Design review of the part built by this model. Coordinates are the model's own, in mm. A direction names the side the tool comes from. Give positions to 0.01 mm unless a question says otherwise; leave off trailing zeros. Write each loop counter-clockwise with the first axis right and the second up, starting at its lowest first coordinate (ties: lowest second). Pieces come first, ordered by that corner, then holes.
```python
from build123d import *

# Parameters (mm, degrees)
F0_W     = 482.6
F0_H     = 50.8
F0_W_2   = 50.8
F0_W_3   = 152.4
F0_H_2   = 101.6
F0_W_4   = 482.6000000003
F0_H_3   = 152.4
F0_W_5   = 381.0000000003
F0_W_6   = 151.9448201656
F0_H_4   = 76.2
F0_W_7   = 51.7103596687
F0_H_5   = 177.8
F0_H_6   = 279.4
F0_W_8   = 380.9999999997
F1_DEPTH = 50.8


with BuildPart() as f1:
    # F0 (on Front) → F1 (new body)
    with BuildSketch(Plane.XZ):
        with Locations((-977.9, 101.6)):
            Rectangle(F0_W, F0_H)
        with Locations((-711.2, 101.6)):
            Rectangle(F0_W_2, F0_H)
        Polygon((-685.8, 76.2), (-736.6, 76.2), (-736.6, -76.2), (-685.8, -76.2), (-685.8, 0), align=None)
        with Locations((-609.6, 101.6)):
            Rectangle(F0_W_3, F0_H)
        with Locations((-711.2, 177.8)):
            Rectangle(F0_W_2, F0_H_2)
        with Locations((-977.9000000001, -101.6)):
            Rectangle(F0_W_4, F0_H)
        with Locations((-711.2, -101.6)):
            Rectangle(F0_W_2, F0_H)
        with Locations((-508, 101.6)):
            Rectangle(F0_W_2, F0_H)
        with Locations((-609.6, -101.6)):
            Rectangle(F0_W_3, F0_H)
        with Locations((-711.2, -177.8)):
            Rectangle(F0_W_2, F0_H_2)
        with Locations((-508, 203.2)):
            Rectangle(F0_W_2, F0_H_3)
        with Locations((-508, -101.6)):
            Rectangle(F0_W_2, F0_H)
        with Locations((-508, 304.8)):
            Rectangle(F0_W_2, F0_H)
        with Locations((-723.9000000001, 304.8)):
            Rectangle(F0_W_5, F0_H)
        with Locations((-508, -203.2)):
            Rectangle(F0_W_2, F0_H_3)
        with Locations((-406.6275899172, 304.8)):
            Rectangle(F0_W_6, F0_H)
        with Locations((-508, 368.3)):
            Rectangle(F0_W_2, F0_H_4)
        with Locations((-723.9000000001, -304.8)):
            Rectangle(F0_W_5, F0_H)
        with Locations((-508, -304.8)):
            Rectangle(F0_W_2, F0_H)
        with Locations((-304.8, 304.8)):
            Rectangle(F0_W_7, F0_H)
        with Locations((-406.6275899172, -304.8)):
            Rectangle(F0_W_6, F0_H)
        with Locations((-508, -368.3)):
            Rectangle(F0_W_2, F0_H_4)
        with Locations((-202.9724100828, 304.8)):
            Rectangle(F0_W_6, F0_H)
        with Locations((-304.8, 419.1)):
            Rectangle(F0_W_7, F0_H_5)
        with Locations((-304.8, -304.8)):
            Rectangle(F0_W_7, F0_H)
        with Locations((-101.6, 304.8)):
            Rectangle(F0_W_2, F0_H)
        with Locations((-202.9724100828, -304.8)):
            Rectangle(F0_W_6, F0_H)
        with Locations((-304.8, -419.1)):
            Rectangle(F0_W_7, F0_H_5)
        Polygon((-76.2, 330.2), (-76.2, 279.4), (-2e-10, 279.4), (76.2, 279.4), (76.2, 330.2), align=None)
        with Locations((-101.6, 469.9)):
            Rectangle(F0_W_2, F0_H_6)
        with Locations((-101.6, -304.8)):
            Rectangle(F0_W_2, F0_H)
        with Locations((101.6, 304.8)):
            Rectangle(F0_W_2, F0_H)
        Polygon((-3e-10, -279.4), (-76.2, -279.4), (-76.2, -330.2), (76.2, -330.2), (76.2, -279.4), align=None)
        with Locations((-101.6, -469.9)):
            Rectangle(F0_W_2, F0_H_6)
        with Locations((203.2, 304.8)):
            Rectangle(F0_W_3, F0_H)
        with Locations((101.6, 469.9)):
            Rectangle(F0_W_2, F0_H_6)
        with Locations((101.6, -304.8)):
            Rectangle(F0_W_2, F0_H)
        with Locations((508, 101.6)):
            Rectangle(F0_W_2, F0_H)
        with Locations((304.8, 304.8)):
            Rectangle(F0_W_2, F0_H)
        with Locations((203.2, -304.8)):
            Rectangle(F0_W_3, F0_H)
        with Locations((101.6, -469.9)):
            Rectangle(F0_W_2, F0_H_6)
        with Locations((609.6, 101.6)):
            Rectangle(F0_W_3, F0_H)
        with Locations((508, 203.2)):
            Rectangle(F0_W_2, F0_H_3)
        with Locations((406.4, 304.8)):
            Rectangle(F0_W_3, F0_H)
        with Locations((304.8, 419.1)):
            Rectangle(F0_W_2, F0_H_5)
        with Locations((508, -101.6)):
            Rectangle(F0_W_2, F0_H)
        with Locations((304.8, -304.8)):
            Rectangle(F0_W_2, F0_H)
        with Locations((711.2, 101.6)):
            Rectangle(F0_W_2, F0_H)
        Polygon((736.6, 76.2), (685.8, 76.2), (685.8, 0), (685.8, -76.2), (736.6, -76.2), align=None)
        with Locations((508, 304.8)):
            Rectangle(F0_W_2, F0_H)
        with Locations((609.6, -101.6)):
            Rectangle(F0_W_3, F0_H)
        with Locations((508, -203.2)):
            Rectangle(F0_W_2, F0_H_3)
        with Locations((406.4, -304.8)):
            Rectangle(F0_W_3, F0_H)
        with Locations((304.8, -419.1)):
            Rectangle(F0_W_2, F0_H_5)
        with Locations((977.9000000001, 101.6)):
            Rectangle(F0_W_4, F0_H)
        with Locations((711.2, 177.8)):
            Rectangle(F0_W_2, F0_H_2)
        with Locations((723.8999999999, 304.8)):
            Rectangle(F0_W_8, F0_H)
        with Locations((508, 368.3)):
            Rectangle(F0_W_2, F0_H_4)
        with Locations((711.2, -101.6)):
            Rectangle(F0_W_2, F0_H)
        with Locations((508, -304.8)):
            Rectangle(F0_W_2, F0_H)
        with Locations((977.9, -101.6)):
            Rectangle(F0_W, F0_H)
        with Locations((711.2, -177.8)):
            Rectangle(F0_W_2, F0_H_2)
        with Locations((723.8999999999, -304.8)):
            Rectangle(F0_W_8, F0_H)
        with Locations((508, -368.3)):
            Rectangle(F0_W_2, F0_H_4)
        with Locations((-304.8, 203.2)):
            Rectangle(F0_W_7, F0_H_3)
        with Locations((-101.6, 203.2)):
            Rectangle(F0_W_2, F0_H_3)
        with Locations((101.6, 203.2)):
            Rectangle(F0_W_2, F0_H_3)
        with Locations((304.8, 203.2)):
            Rectangle(F0_W_2, F0_H_3)
        Polygon((330.2, 76.2), (279.4, 76.2), (279.4, 0), (304.8, 0), (330.2, 0), align=None)
        Polygon((304.8, 0), (279.4, 0), (279.4, -76.2), (330.2, -76.2), (330.2, 0), align=None)
        with Locations((304.8, -101.6)):
            Rectangle(F0_W_2, F0_H)
        with Locations((304.8, -203.2)):
            Rectangle(F0_W_2, F0_H_3)
        with Locations((304.8, 101.6)):
            Rectangle(F0_W_2, F0_H)
        Polygon((533.4, 76.2), (482.6, 76.2), (482.6, 0), (508, 0), (533.4, 0), align=None)
        Polygon((508, 0), (482.6, 0), (482.6, -76.2), (533.4, -76.2), (533.4, 0), align=None)
        with Locations((101.6, -203.2)):
            Rectangle(F0_W_2, F0_H_3)
        with Locations((101.6, -101.6)):
            Rectangle(F0_W_2, F0_H)
        Polygon((101.6, 0), (76.2, 0), (76.2, -76.2), (127, -76.2), (127, 0), align=None)
        Polygon((127, 76.2), (76.2, 76.2), (76.2, 0), (101.6, 0), (127, 0), align=None)
        with Locations((101.6, 101.6)):
            Rectangle(F0_W_2, F0_H)
        with Locations((-101.6, 101.6)):
            Rectangle(F0_W_2, F0_H)
        Polygon((-76.2, 76.2), (-127, 76.2), (-127, 0), (-101.6, 0), (-76.2, 0), align=None)
        Polygon((-101.6, 0), (-127, 0), (-127, -76.2), (-76.2, -76.2), (-76.2, 0), align=None)
        with Locations((-101.6, -101.6)):
            Rectangle(F0_W_2, F0_H)
        with Locations((-101.6, -203.2)):
            Rectangle(F0_W_2, F0_H_3)
        with Locations((-304.8, -203.2)):
            Rectangle(F0_W_7, F0_H_3)
        with Locations((-304.8, -101.6)):
            Rectangle(F0_W_7, F0_H)
        Polygon((-304.8, 0), (-330.6551798344, 0), (-330.6551798344, -76.2), (-278.9448201656, -76.2), (-278.9448201656, 0), align=None)
        Polygon((-278.9448201656, 76.2), (-330.6551798344, 76.2), (-330.6551798344, 0), (-304.8, 0), (-278.9448201656, 0), align=None)
        with Locations((-304.8, 101.6)):
            Rectangle(F0_W_7, F0_H)
        Polygon((-482.6, 76.2), (-533.4, 76.2), (-533.4, 0), (-508, 0), (-482.6, 0), align=None)
        Polygon((-508, 0), (-533.4, 0), (-533.4, -76.2), (-482.6, -76.2), (-482.6, 0), align=None)
        with Locations((-406.6275899172, 101.6)):
            Rectangle(F0_W_6, F0_H)
        with Locations((-202.9724100828, 101.6)):
            Rectangle(F0_W_6, F0_H)
        Polygon((-76.2, 127), (-76.2, 76.2), (76.2, 76.2), (76.2, 127), (0, 127), align=None)
        with Locations((203.2, 101.6)):
            Rectangle(F0_W_3, F0_H)
        with Locations((406.4, 101.6)):
            Rectangle(F0_W_3, F0_H)
        with Locations((406.4, -101.6)):
            Rectangle(F0_W_3, F0_H)
        with Locations((203.2, -101.6)):
            Rectangle(F0_W_3, F0_H)
        Polygon((76.2, -76.2), (-76.2, -76.2), (-76.2, -127), (-3e-10, -127), (76.2, -127), align=None)
        with Locations((-202.9724100828, -101.6)):
            Rectangle(F0_W_6, F0_H)
        with Locations((-406.6275899172, -101.6)):
            Rectangle(F0_W_6, F0_H)
    extrude(amount=F1_DEPTH)


solid = f1.part
```
(1) Consider section C-C, the plane x = -609. Give the boundary of the cut face in (y, z).
Resolved:
outline: (-50.8, -330.2) - (0, -330.2) - (0, -279.4) - (-50.8, -279.4) - close; (-50.8, -127) - (0, -127) - (0, -76.2) - (-50.8, -76.2) - close; (-50.8, 76.2) - (0, 76.2) - (0, 127) - (-50.8, 127) - close; (-50.8, 279.4) - (0, 279.4) - (0, 330.2) - (-50.8, 330.2) - close
(2) Clearance check with flat-ended pins moving along their axes: P1, Ø10, axis at y = -8.5, z = 393, coming from the -X side; P2, Ø5, axis at y = -39.5, z = -2, coming from the +X side; P3, Ø5, axis at x = -313.5, y = -15.5, coming from the -Z side. State where each tip first meets the part, or that it passes through.
Resolved:
P1: stops at x = -533.4
P2: stops at x = 736.6
P3: stops at z = -508
(3) Tool access review of faces 1 (the face through (736.6, -25, -1)), 2 (the face through (127, -25, 468)), 3 (the face through (-482.6, -25, -369)), 4 (the face through (1, -25, -76.2)), 5 (the face through (533.4, -25, -369)): name each direction out of +Z, -Z, +X, -X, +Y, -Y from which nothing blocks a thin tool from reaching the whole face with its end or side.
Resolved:
face 1: +X, +Y, -Y
face 2: +Z, +Y, -Y
face 3: -Z, +Y, -Y
face 4: +Y, -Y
face 5: -Z, +X, +Y, -Y
(4) Mouldability with a two-part tool opening along X and no side actions: class faces 6 (the face through (-736.6, -25, -179)), 7 (the face through (-975, -25, 127)), 8 (the face through (-127, -25, -202)) as pulls with the +X half, pulls with the -X half, needs draft (parallel to the pull), parting line crosses it, or undercut.
Resolved:
face 6: pulls with the -X half
face 7: needs draft
face 8: undercut
(5) To check wall thickness, follow L1, parallel to X at y = -40, z = 415; L2, parallel to Z at x = -367, y = -36; L3, parallel to Z at x = 714, y = -47.5. State the ranges of each line that lie inside material, in increasing order.
Resolved:
L1: x = -330.66 to -278.94, -127 to -76.2, 76.2 to 127, 279.4 to 330.2
L2: z = -330.2 to -279.4, -127 to -76.2, 76.2 to 127, 279.4 to 330.2
L3: z = -330.2 to -279.4, -228.6 to 228.6, 279.4 to 330.2
(6) Consider section D-D, the plane z = -530. Give the boundary of the cut face in (x, y), then the cut area to 3 significant figures.
Resolved:
outline: (-127, -50.8) - (-76.2, -50.8) - (-76.2, 0) - (-127, 0) - close; (76.2, -50.8) - (127, -50.8) - (127, 0) - (76.2, 0) - close
area: 5,160 mm2
(7) Consider section A-A, the plane x = -1054. Give the boundary of the cut face in (y, z).
Resolved:
outline: (-50.8, -127) - (0, -127) - (0, -76.2) - (-50.8, -76.2) - close; (-50.8, 76.2) - (0, 76.2) - (0, 127) - (-50.8, 127) - close
(8) Consider section B-B, the plane z = 374.5. Give the boundary of the cut face in (x, y), then the cut area to 3 significant figures.
Resolved:
outline: (-533.4, -50.8) - (-482.6, -50.8) - (-482.6, 0) - (-533.4, 0) - close; (-330.66, -50.8) - (-278.94, -50.8) - (-278.94, 0) - (-330.66, 0) - close; (-127, -50.8) - (-76.2, -50.8) - (-76.2, 0) - (-127, 0) - close; (76.2, -50.8) - (127, -50.8) - (127, 0) - (76.2, 0) - close; (279.4, -50.8) - (330.2, -50.8) - (330.2, 0) - (279.4, 0) - close; (482.6, -50.8) - (533.4, -50.8) - (533.4, 0) - (482.6, 0) - close
area: 15,500 mm2
